Design review of the part built by this model. Coordinates are the model's own, in mm. A direction names the side the tool comes from. Give positions to 0.01 mm unless a question says otherwise; leave off trailing zeros. Order: outer loops, then holes, each group sorted by start corner. A loop starts at its lowest first (then second) coordinate and runs counter-clockwise, first axis right, second up. Notation, with made-up numbers: (18, 43) -> (66, 43) arc R17 cw to (66, 57) -> close; hole circle Ø5 at (71, -40). An arc over 180 degrees is marked (long way). One line per item, written item: value.
from build123d import *

# Parameters (mm, degrees)
SKETCH1_W           = 38.699948
SKETCH1_H           = 153.19375
BOSS_EXTRUDE1_DEPTH = 2.54
BOSS_EXTRUDE2_DEPTH = 23.706666582
CUT_EXTRUDE1_DEPTH  = 160.77490754


with BuildPart() as part:
    # Sketch1 → Boss-Extrude1 (new body)
    with BuildSketch(Plane(origin=(0, 0, 0), x_dir=(1, 0, 0), z_dir=(0, 1, 0))):
        with Locations((19.349974, 76.596875)):
            Rectangle(SKETCH1_W, SKETCH1_H)
    extrude(amount=BOSS_EXTRUDE1_DEPTH)

    # Sketch3 → Boss-Extrude2 (add)
    with BuildSketch(Plane(origin=(0, 2.54, 0), x_dir=(1, 0, 0), z_dir=(0, 1, 0))):
        Polygon((6.35, 146.84375), (14.5875, 146.84375), (14.5875, 143.66875), (19.35, 143.66875), (32.35, 141.684375), (32.35, 135.41375), (38.7, 135.41375), (38.7, 153.19375), (0, 153.19375), (0, 135.41375), (6.35, 135.41375), align=None)
        Polygon((17.7625, 9.525), (14.5875, 9.525), (14.5875, 6.35), (6.35, 6.35), (6.35, 17.78), (0, 17.78), (0, 0), (30.703239638, 0), (30.703239638, 16.115739638), (24.353239638, 16.115739638), align=None)
    extrude(amount=BOSS_EXTRUDE2_DEPTH)

    # Sketch4 → Cut-Extrude1 (cut, through all)
    with BuildSketch(Plane(origin=(0, 2.54, 0), x_dir=(1, 0, 0), z_dir=(0, 1, 0))):
        Polygon((30.703239638, 0), (38.699948, 0), (38.699948, 135.41375), (30.703239638, 16.115739638), align=None)
    extrude(amount=-CUT_EXTRUDE1_DEPTH, mode=Mode.SUBTRACT)


solid = part.part
Item 1: Add section B-B on x = 3. Give the boundary of the cut face in (y, z), plus the area to 3 significant figures.
Returned:
outline: (0, -153.19) -> (26.25, -153.19) -> (26.25, -135.41) -> (2.54, -135.41) -> (2.54, -17.78) -> (26.25, -17.78) -> (26.25, 0) -> (0, 0) -> close
area: 1,230 mm²
Item 2: Machinability: for faces 5 (the flat face through (11, 14, -6.35)), 6 (the flat face through (30.703, 13, -8)), 7 (the flat face through (35, 14, -135.414)), 8 (the flat face through (15, 13, 0)), which of the approach directions +Z, -Z, +X, -X, +Y, -Y give a long, thin tool a straight path to every point of the face, cutting with its end or side? Answer none if there is none.
Returned:
face 5: +Y
face 6: +Z, +X, +Y, -Y
face 7: +Z, +X, -X, +Y
face 8: +Z, +X, -X, +Y, -Y
Item 3: Add section C-C on z = -13.5. Give the boundary of the cut face in (x, y).
Returned:
outline: (0, 0) -> (30.7, 0) -> (30.7, 26.25) -> (21.74, 26.25) -> (21.74, 2.54) -> (6.35, 2.54) -> (6.35, 26.25) -> (0, 26.25) -> close
Item 4: Clearance check with flat-ended pins moving along their axes: P1, Ø5, axis at y = 19.5, z = -8.5, coming from the +X side; P2, Ø5, axis at x = 34.5, y = 16, coming from the +Z side; P3, Ø4, axis at x = 4.5, z = -24, coming from the +Y side. State where each tip first meets the part, or that it passes through.
Returned:
P1: x = 30.7
P2: z = -135.41
P3: y = 2.54
Item 5: Add section D-D on x = 34. Give the boundary of the cut face in (y, z).
Returned:
outline: (0, -153.19) -> (26.25, -153.19) -> (26.25, -135.41) -> (2.54, -135.41) -> (2.54, -65.3) -> (0, -65.3) -> close
Item 6: Draft analysis for pull direction Z (two halves, no side actions). For faces 1 (the flat face through (6.35, 14, -12)), 2 (the flat face through (19, 0, -78)), 3 (the flat face through (14.588, 14, -8)), 4 (the flat face through (34.758, 1.288, -76.6)), state which applies: pulls with the +Z half, pulls with the -Z half, needs draft (parallel to the pull), parting line crosses it, or undercut.
Returned:
face 1: undercut
face 2: needs draft
face 3: undercut
face 4: pulls with the +Z half
Item 7: To check wall thickness, follow line 1 along Z through (x, y) = (11, 10.75); line 2 along Z through (x, y) = (6, 4); line 3 along X through (y, z) = (22.75, -6.5). State the ranges of each line that lie inside material, in increasing order. Write a range as from..to.
Returned:
line 1: -153.19..-146.84, -6.35..0
line 2: -153.19..-135.41, -17.78..0
line 3: 0..6.35, 14.59..30.7
